Geometry: see drawing. Coordinates: mm, zero at the bounding-box minimum. A direction names the side the tool comes from. Round coordinates to 2 decimals unless told otherwise and drop trailing zeros. Write each loop counter-clockwise with the first axis right and the second up, starting at its lowest first coordinate (ties: lowest second). Pieces come first, ordered by that corner, then holes.
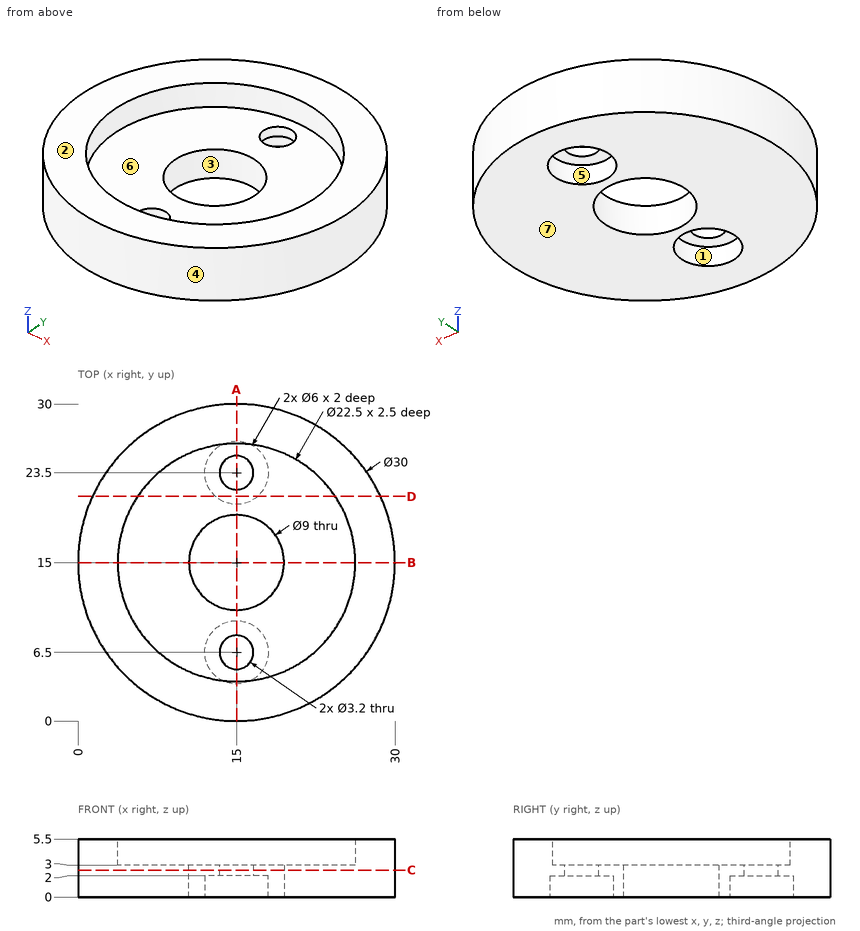
1) Section query B-B on y = 15. Return the cut outline in (x, z), then the cut area to 4 significant figures.
Taken from the geometry:
outline: (0, 0) - (10.5, 0) - (10.5, 3) - (3.75, 3) - (3.75, 5.5) - (0, 5.5) - close; (19.5, 0) - (30, 0) - (30, 5.5) - (26.25, 5.5) - (26.25, 3) - (19.5, 3) - close
area: 81.75 mm2
2) Reachability of the marked faces 5, 6 and 7 from +Z, -Z, +X, -X, +Y, -Y: full face, straight path, thin tool, end or side. Return the list, or none.
Taken from the geometry:
face 5: -Z
face 6: +Z
face 7: -Z, +X, -X, +Y, -Y
3) Contact query for flat-ended pins moving along their axis: P1, Ø3, axis at x = 19.5, z = 2.5, coming from the +Y side; P2, Ø8, axis at x = 18.5, y = 14, coming from the +Z side; P3, Ø1, axis at y = 7.5, z = 4.5, coming from the -X side. Output: stop coordinate, or through.
Taken from the geometry:
P1: stops at y = 29.7
P2: stops at z = 3
P3: stops at x = 1.73
4) Material intervals for line 1 (Y direction, x = 15, z = 2.7); line 2 (Y direction, x = 15, z = 0.65); line 3 (Y direction, x = 15, z = 4.55), sorted ascending.
Taken from the geometry:
line 1: y = 0 to 4.9, 8.1 to 10.5, 19.5 to 21.9, 25.1 to 30
line 2: y = 0 to 3.5, 9.5 to 10.5, 19.5 to 20.5, 26.5 to 30
line 3: y = 0 to 3.75, 26.25 to 30
5) Pull-direction query (X, two-part tool) for the marked faces 1, 2, 3 and 4; classes: released by +X, released by -X, zero draft, split by the parting line, or undercut.
Taken from the geometry:
face 1: undercut
face 2: zero draft
face 3: undercut
face 4: split by the parting line
6) Section query A-A on x = 15. Return the cut outline in (y, z).
Taken from the geometry:
outline: (0, 0) - (3.5, 0) - (3.5, 2) - (4.9, 2) - (4.9, 3) - (3.75, 3) - (3.75, 5.5) - (0, 5.5) - close; (8.1, 2) - (9.5, 2) - (9.5, 0) - (10.5, 0) - (10.5, 3) - (8.1, 3) - close; (19.5, 0) - (20.5, 0) - (20.5, 2) - (21.9, 2) - (21.9, 3) - (19.5, 3) - close; (25.1, 2) - (26.5, 2) - (26.5, 0) - (30, 0) - (30, 5.5) - (26.25, 5.5) - (26.25, 3) - (25.1, 3) - close
7) Section query D-D on y = 21.25. Return the cut outline in (x, z), then the cut area to 3 significant figures.
Taken from the geometry:
outline: (1.36, 0) - (13.02, 0) - (13.02, 2) - (16.98, 2) - (16.98, 0) - (28.64, 0) - (28.64, 5.5) - (24.35, 5.5) - (24.35, 3) - (5.65, 3) - (5.65, 5.5) - (1.36, 5.5) - close
area: 95.3 mm2
8) Section query C-C on z = 2.55. Return the cut outline in (x, y), then the cut area to 3 significant figures.
Taken from the geometry:
outline: circle Ø30 at (15, 15); hole circle Ø9 at (15, 15); hole circle Ø3.2 at (15, 6.5); hole circle Ø3.2 at (15, 23.5)
area: 627 mm2
